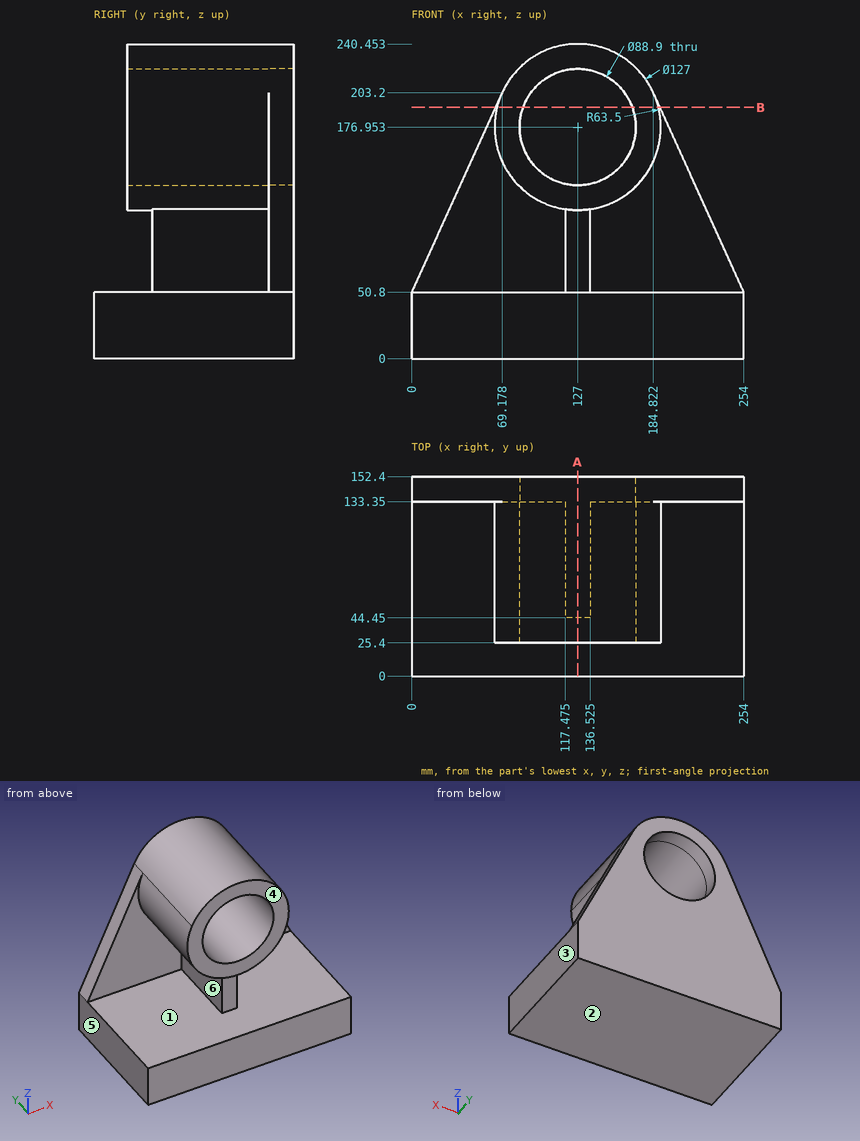
Could you check a few things on this drawing? It's one solid part, dimensions in mm from its lowest x, y, z. A direction names the side the tool comes from. Round coordinates to 2 decimals unless told otherwise and drop trailing zeros. Loops run counter-clockwise (first coordinate to the right, second up) from the corner with the lowest first, then second, coordinate; pieces in that order, holes last.
Q1. Please list where these lines run through material, in increasing order: L1, parallel to Z at x = 127, y = 108; L2, parallel to Z at x = 105.5, y = 111.5; L3, parallel to X at y = 92.5, z = 179.5.
Q2. Thinking about a two-plate mould opening in Z: for the marked faces 1, 2 and 3, which applies, pulls with the +Z half, pulls with the -Z half, needs draft (parallel to the pull), parting line crosses it, or undercut?
Q3. On a 3-axis mill with a long thin cutter (end or side, diameter ignored), from which of +Z, -Z, +X, -X, +Y, -Y can I reach the whole of each face in a straight line? I mean the marked faces 4, 5 and 6. Say none if no direction works.
Q4. I want a section at A-A (x = 127). Write out the boundary of the cut face in (y, z), and give its area (3 significant figures).
Q5. I want a section at B-B (z = 192). Write out the boundary of the cut face in (x, y), and give its area (3 significant figures).
Q6. For P1, Ø1.5, axis at x = 61.5, y = 135.5, coming from the -Z side; P2, Ø8, axis at y = 95.5, z = 108.5, coming from the +X side (3 decimals); P3, Ø5.5, axis at x = 124.5, z = 72.5, coming from the -Y side; P4, Ø6, axis at y = 31.5, z = 124, coming from the +X side, each with a flat end and sliding along its axis, tell me the tip position at first contact or that it passes through.
Answer below:
1. L1: z = 0 to 132.5, 221.4 to 240.45
1. L2: z = 0 to 50.8, 117.2 to 138.05, 215.86 to 236.7
1. L3: x = 63.55 to 82.62, 171.38 to 190.45
2. face 1: undercut
2. face 2: pulls with the -Z half
2. face 3: needs draft
3. face 4: +Z, +X, -X, -Y
3. face 5: +Z, -Z, -X, +Y, -Y
3. face 6: -X, -Y
4. outline: (0, 0) - (152.4, 0) - (152.4, 132.5) - (25.4, 132.5) - (25.4, 113.45) - (44.45, 113.45) - (44.45, 50.8) - (0, 50.8) - close; (25.4, 221.4) - (152.4, 221.4) - (152.4, 240.45) - (25.4, 240.45) - close
4. area: 19,300 mm2
5. outline: (64.09, 133.35) - (65.31, 133.35) - (65.31, 25.4) - (85.17, 25.4) - (85.17, 152.4) - (64.09, 152.4) - close; (168.83, 25.4) - (188.69, 25.4) - (188.69, 133.35) - (189.91, 133.35) - (189.91, 152.4) - (168.83, 152.4) - close
5. area: 5,090 mm2
6. P1: stops at z = 0
6. P2: stops at x = 136.525
6. P3: stops at y = 44.45
6. P4: stops at x = 166.2
